Check sheet for the modelled part. Datum: model origin and axes. Units: mm. Face numbers are marked on the shaded views. A direction names the side the tool comes from. Give positions to 0.01 mm unless a question says otherwise; leave off trailing zeros. Order: outer loops, then holes, each group sorted by start corner. A loop starts at its lowest first (then second) coordinate and runs counter-clockwise, first axis right, second up.
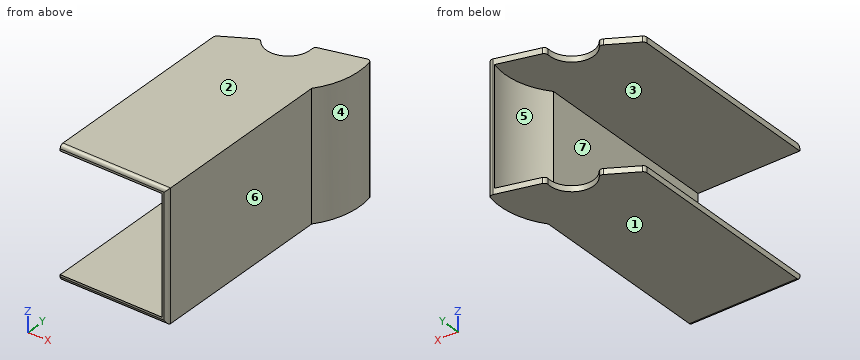
```python
from build123d import *

# Parameters (mm, degrees)
SKETCH1_R               = 49
BOSS_EXTRUDE1_DEPTH     = 88
CUT_EXTRUDE1_DEPTH      = 88
SKETCH3_W               = 77.94
SKETCH3_H               = 128.535806693
BOSS_EXTRUDE2_DEPTH     = 88
CUT_EXTRUDE2_DEPTH      = 40.1
CUT_EXTRUDE2_DEPTH_BACK = 40.1
SKETCH4_R               = 45.5
CUT_EXTRUDE3_DEPTH      = 40.1
CUT_EXTRUDE3_DEPTH_BACK = 40.1
SKETCH5_W               = 69.94
SKETCH5_H               = 158.24
CUT_EXTRUDE5_DEPTH      = 202.302306246
CUT_EXTRUDE5_DEPTH_BACK = 4
SKETCH6_W               = 88
SKETCH6_H               = 170.045451323
SKETCH7_R               = 15
CUT_EXTRUDE6_DEPTH      = 188.576378044
FILLET1_R               = 2.5


with BuildPart() as part:
    # Sketch1 → Boss-Extrude1 (new body)
    with BuildSketch(Plane.XY):
        Circle(SKETCH1_R)
    extrude(amount=BOSS_EXTRUDE1_DEPTH)

    # Sketch2 → Cut-Extrude1 (cut)
    with BuildSketch(Plane(origin=(0, 0, 0), x_dir=(-1, 0, 0), z_dir=(0, 0, -1))):
        with BuildLine():
            Line((0, 0), (-47.330365488, 12.68213321))
            ThreePointArc((-47.330365488, 12.68213321), (18.751488186, 45.270097093), (42.435244785, -24.5))
            Line((42.435244785, -24.5), (0, 0))
        make_face()
    extrude(amount=-CUT_EXTRUDE1_DEPTH, mode=Mode.SUBTRACT)

    # Sketch3 → Boss-Extrude2 (add)
    with BuildSketch(Plane(origin=(0, 0, 0), x_dir=(-1, 0, 0), z_dir=(0, 0, -1))):
        with Locations((0, -93.972096654)):
            Rectangle(SKETCH3_W, SKETCH3_H)
    extrude(amount=-BOSS_EXTRUDE2_DEPTH)

    # Sketch4 → Cut-Extrude2 (cut, two sides: drawn at the far end of the back side and taken through both)
    with BuildSketch(Plane(origin=(0, 0, 44), x_dir=(-1, 0, 0), z_dir=(0, 0, -1)).offset(-CUT_EXTRUDE2_DEPTH_BACK)):
        Circle(SKETCH4_R)
    extrude(amount=CUT_EXTRUDE2_DEPTH + CUT_EXTRUDE2_DEPTH_BACK, mode=Mode.SUBTRACT)

    # Sketch5 → Cut-Extrude3 (cut, two sides: drawn at the far end of the back side and taken through both)
    with BuildSketch(Plane(origin=(0, 0, 44), x_dir=(-1, 0, 0), z_dir=(0, 0, -1)).offset(-CUT_EXTRUDE3_DEPTH_BACK)):
        with Locations((0, -79.12)):
            Rectangle(SKETCH5_W, SKETCH5_H)
    extrude(amount=CUT_EXTRUDE3_DEPTH + CUT_EXTRUDE3_DEPTH_BACK, mode=Mode.SUBTRACT)

    # Sketch6 → Cut-Extrude5 (cut, two sides: drawn at the far end of the back side and taken through both)
    with BuildSketch(Plane.ZY.offset(38.97).offset(-CUT_EXTRUDE5_DEPTH_BACK)):
        with Locations((44, -73.246459109)):
            Rectangle(SKETCH6_W, SKETCH6_H)
    extrude(amount=CUT_EXTRUDE5_DEPTH + CUT_EXTRUDE5_DEPTH_BACK, mode=Mode.SUBTRACT)

    # Sketch7 → Cut-Extrude6 (cut, through all)
    with BuildSketch(Plane(origin=(0, 0, 0), x_dir=(-1, 0, 0), z_dir=(0, 0, -1))):
        Circle(SKETCH7_R)
    extrude(amount=-CUT_EXTRUDE6_DEPTH, mode=Mode.SUBTRACT)

    # Fillet1
    fillet1_edges = [part.edges().sort_by_distance(p)[0] for p in [
        (47.330365488, 12.68213321, 44),
        (14.488887394, 3.882285677, 86.05),
        (14.488887394, 3.882285677, 1.95),
        (-12.990381057, -7.5, 1.95),
        (-12.990381057, -7.5, 86.05),
        (2, -158.24, 0),
        (38.97, -158.24, 44),
        (2, -158.24, 88),
        (-34.97, -20.189938914, 1.95),
        (-34.97, -20.189938914, 86.05),
    ]]
    fillet(fillet1_edges, radius=FILLET1_R)


solid = part.part
```
Q1. Sectioned sample at B-B, the plane y = -124.5. Record the cut outline in (x, z), plus the area to 3 significant figures.
Q2. Sectioned sample at C-C, the plane x = 2.5. Record the cut outline in (y, z), plus the area to 3 significant figures.
Q3. Sectioned sample at A-A, the plane x = -9. Record the cut outline in (y, z), plus the area to 3 significant figures.
Q4. Tool access check on the marked faces 5, 6 and 7. Record the directions out of +Z, -Z, +X, -X, +Y, -Y that give a thin tool (end or side, any length) a straight path to the whole face; none if there is none.
Q5. Material ranges on line 1 (Z direction, x = 11, y = -41); line 2 (X direction, y = 0.5, z = 62); line 3 (X direction, y = -112.5, z = 35), recorded low to high.
Q6. Go/stop test with flat-tipped pins: P1, Ø5, axis at y = -90, z = 67, coming from the +X side; P2, Ø1.5, axis at y = -15.5, z = 40.5, coming from the +X side. Record where each tip stops, or that it passes through.
Q7. Sectioned sample at D-D, the plane z = 79. Record the cut outline in (x, y), plus the area to 3 significant figures.
Q8. Draft check along Z on the marked faces 1, 2, 3 and 4. Enter one of: pulls with the +Z half, pulls with the -Z half, needs draft (parallel to the pull), parting line crosses it, or undercut.
Filled in:
1. outline: (-34.97, 0) - (38.97, 0) - (38.97, 88) - (-34.97, 88) - (-34.97, 84.1) - (34.97, 84.1) - (34.97, 3.9) - (-34.97, 3.9) - close
1. area: 898 mm2
2. outline: (-158.24, 2.5) arc R2.5 ccw to (-155.74, 0) - (-14.79, 0) - (-14.79, 3.9) - (-158.24, 3.9) - close; (-158.24, 84.1) - (-14.79, 84.1) - (-14.79, 88) - (-155.74, 88) arc R2.5 ccw to (-158.24, 85.5) - close
2. area: 1,120 mm2
3. outline: (-158.24, 2.5) arc R2.5 ccw to (-155.74, 0) - (-12, 0) - (-12, 3.9) - (-158.24, 3.9) - close; (-158.24, 84.1) - (-12, 84.1) - (-12, 88) - (-155.74, 88) arc R2.5 ccw to (-158.24, 85.5) - close
3. area: 1,140 mm2
4. face 5: -X
4. face 6: +Z, -Z, +X, -Y
4. face 7: -X, +Y, -Y
5. line 1: z = 0 to 3.9, 84.1 to 88
5. line 2: x = 45.5 to 49
5. line 3: x = 34.97 to 38.97
6. P1: stops at x = 38.97
6. P2: stops at x = 46.73
7. outline: (34.97, -158.24) - (36.47, -158.24) arc R2.5 ccw to (38.97, -155.74) - (38.97, -29.7) arc R49 ccw to (47.94, 10.12) arc R2.5 ccw to (44.85, 12.02) - (43.95, 11.78) arc R45.5 cw to (34.97, -29.11) - close
7. area: 667 mm2
8. face 1: pulls with the -Z half
8. face 2: pulls with the +Z half
8. face 3: undercut
8. face 4: needs draft
